Can you work these out from the model? Positions are in its coordinate system, mm. A direction names the side the tool comes from. Round coordinates to 2 decimals unless told otherwise and drop trailing zeros. Write each loop counter-clockwise with the first axis right and the second up, starting at its lowest first coordinate (ties: lowest second). Pieces come first, ordered by that corner, then holes. Notation, with made-up numbers: M 63,45.25 L 109,45.25 A28 cw 109,76.25 Z; hole C 88,-24.5 d11. An arc over 180 degrees is marked long. Answer as a JSON object with one key per item and string values. Group by question number.
1) Suppose I cut it at C-C, the plane y = -10. Write out the boundary of the cut face in (x, z), and give its area (3 significant figures).
2) Suppose I cut it at D-D, the plane z = 6.75. Write out the boundary of the cut face in (x, y).
3) Please list where these lines run through material, in increasing order: L1, parallel to X at y = -11, z = 0.75; L2, parallel to Y at x = -7.5, z = 13.25; L3, parallel to Y at x = -22.5, z = 1.6. Write a range as [from, to].
4) Suppose I cut it at B-B, the plane z = 14. Write out the boundary of the cut face in (x, y).
5) If we mould it in two halves opening along Y, with no side actions, what happens to faces 4 (the flat face through (-15, 0, 7)), 5 (the flat face through (-28, -7, 15)), 6 (the cylindrical face through (-4.64, -9.1, 10.44)), 7 (the flat face through (-39.89, -17.37, 7.4))? For each: +Y half, -Y half, draft (parallel to the pull), parting line (faces both ways), or undercut.
6) On a 3-axis mill with a long thin cutter (end or side, diameter ignored), from which of +Z, -Z, +X, -X, +Y, -Y can I reach the whole of each face in a straight line? I mean faces 1 (the flat face through (-48, -5, 2)), 2 (the flat face through (-25, -12, 6)), 3 (the flat face through (-15, -20, 7)). Say none if no direction works.
7) Suppose I cut it at A-A, the plane x = -22.5. Write out the boundary of the cut face in (y, z), and give its area (3 significant figures).
8) I'm going to push flat-ended pins straight in: pin 1 Ø1.5 at (x, z) = (-25.5, 12) entering from +Y; pin 2 Ø4 at (y, z) = (0.5, 6.5) entering from -X; pin 3 Ø3 at (y, z) = (-1, 7) entering from -X. Where does each tip first touch, or does it pass through?
from build123d import *

# Parameters (mm, degrees)
SKETCH_1_R          = 3
EXTRUDE_1_DEPTH     = 15
SKETCH_4_R          = 5
CUT_EXTRUDE_3_DEPTH = 6
SKETCH_8_R          = 4
CUT_EXTRUDE_4_DEPTH = 3
SKETCH_10_R         = 2.5
CUT_EXTRUDE_5_DEPTH = 10


with BuildPart() as part:
    # 草图1 → 凸台-拉伸1 (new body)
    with BuildSketch(Plane.XY):
        with BuildLine():
            Line((-30, 0), (0, 0))
            Line((0, 0), (0, -20))
            Line((0, -20), (-30, -20))
            Line((-30, -20), (-50.06938155, -14.664278475))
            ThreePointArc((-50.06938155, -14.664278475), (-57.106051537, -2.220832162), (-44.512363219, 4.543271266))
            Line((-44.512363219, 4.543271266), (-30, 0))
        make_face()
        with Locations((-22.5, -10)):
            Circle(SKETCH_1_R, mode=Mode.SUBTRACT)
        with Locations((-7.5, -10)):
            Circle(SKETCH_1_R, mode=Mode.SUBTRACT)
    extrude(amount=EXTRUDE_1_DEPTH)

    # 草图4 → 切除-拉伸3 (cut)
    with BuildSketch(Plane(origin=(0, 0, 0), x_dir=(-1, 0, 0), z_dir=(0, 0, -1))):
        with Locations((7.5, -10)):
            Circle(SKETCH_4_R)
        with Locations((22.5, -10)):
            Circle(SKETCH_4_R)
    extrude(amount=-CUT_EXTRUDE_3_DEPTH, mode=Mode.SUBTRACT)

    # 草图8 → 切除-拉伸4 (cut)
    with BuildSketch(Plane.XY.offset(15)):
        with Locations((-47.5, -5)):
            Circle(SKETCH_8_R)
    extrude(amount=-CUT_EXTRUDE_4_DEPTH, mode=Mode.SUBTRACT)

    # 草图10 → 切除-拉伸5 (cut)
    with BuildSketch(Plane.XY.offset(12)):
        with Locations((-47.5, -5)):
            Circle(SKETCH_10_R)
    extrude(amount=-CUT_EXTRUDE_5_DEPTH, mode=Mode.SUBTRACT)


solid = part.part
Results:
{
 "1": {"outline": "M -56.16,0 L -27.5,0 L -27.5,6 L -25.5,6 L -25.5,15 L -56.16,15 Z; M -19.5,6 L -17.5,6 L -17.5,0 L -12.5,0 L -12.5,6 L -10.5,6 L -10.5,15 L -19.5,15 Z; M -4.5,6 L -2.5,6 L -2.5,0 L 0,0 L 0,15 L -4.5,15 Z", "area": "614 mm^2"},
 "2": {"outline": "M -50.07,-14.66 L -30,-20 L 0,-20 L 0,0 L -30,0 L -44.51,4.54 A10 ccw long Z; hole C -47.5,-5 d5; hole C -22.5,-10 d6; hole C -7.5,-10 d6"},
 "3": {"L1": "[-55.5, -27.4], [-17.6, -12.4], [-2.6, 0]", "L2": "[-20, -13], [-7, 0]", "L3": "[-20, -15], [-5, 0]"},
 "4": {"outline": "M -50.07,-14.66 L -30,-20 L 0,-20 L 0,0 L -30,0 L -44.51,4.54 A10 ccw long Z; hole C -47.5,-5 d8; hole C -22.5,-10 d6; hole C -7.5,-10 d6"},
 "5": {"face 4": "+Y half", "face 5": "draft", "face 6": "undercut", "face 7": "-Y half"},
 "6": {"face 1": "+Z", "face 2": "-Z", "face 3": "+Z, -Z, +X, -X, -Y"},
 "7": {"outline": "M -20,0 L -15,0 L -15,6 L -13,6 L -13,15 L -20,15 Z; M -7,6 L -5,6 L -5,0 L 0,0 L 0,15 L -7,15 Z", "area": "186 mm^2"},
 "8": {"pin 1": "y = 0", "pin 2": "x = -56.87", "pin 3": "x = -57.18"}
}
